The listing builds one solid part. Answer for the finished solid, in the listing's coordinates (mm). Face numbers are marked on the shaded views. A direction names the side the tool comes from. Give positions to 0.01 mm unless a question says otherwise; leave off trailing zeros. Write each loop counter-clockwise with the first axis right and the second up, starting at its lowest first coordinate (ties: lowest second). Pieces come first, ordered by that corner, then holes. Notation, with made-up numbers: (38, 69.5) - (97, 69.5) arc R8 ccw to (97, 79.5) - close; hole circle Ø2 at (45, 83.25). An arc over 180 degrees is marked (long way). Answer in a Markdown table with one row per item. Add a question column.
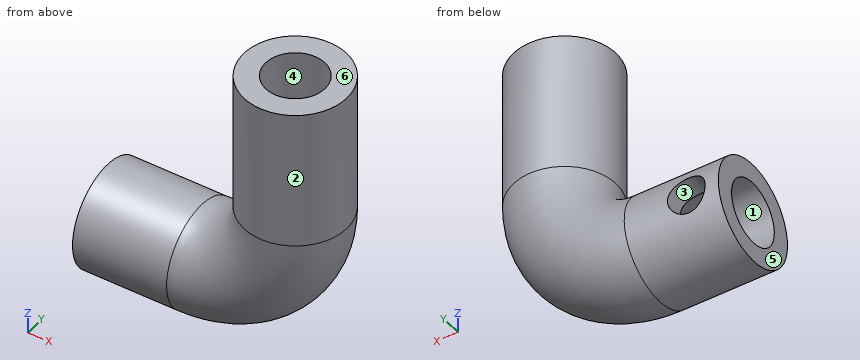
from build123d import *

# Parameters (mm, degrees)
SKETCH4_R         = 5.5
SKETCH6_R         = 3.175
HOLE_SHAFT_DEPTH  = 10
SKETCH7_R         = 3.4
HOLE_POT_DEPTH    = 10
SKETCH8_R         = 2
HOLE_INSERT_DEPTH = 6.5000001
SLOT_BOSS_DEPTH   = 1


with BuildPart() as part:
    # Sweep2: sweep along a path in PROFILE
    with BuildLine(Plane(origin=(0, 0, 0), x_dir=(1, 0, 0), z_dir=(0, 1, 0))) as sweep2_path:
        Line((2.5, -25), (2.5, -10))
        ThreePointArc((2.5, -10), (-0.428932188, -2.928932188), (-7.5, 0))
        Line((-7.5, 0), (-17.5, 0))
    # Sketch4 → Sweep2 (sweep)
    with BuildSketch(Plane.XY.offset(25)):
        with Locations((2.5, 0)):
            Circle(SKETCH4_R)
    sweep(path=sweep2_path.line)

    # Sketch6 → HOLE_SHAFT (cut)
    with BuildSketch(Plane.XY.offset(25)):
        with Locations((2.5, 0)):
            Circle(SKETCH6_R)
    extrude(amount=-HOLE_SHAFT_DEPTH, mode=Mode.SUBTRACT)

    # Sketch7 → HOLE_POT (cut)
    with BuildSketch(Plane.ZY.offset(17.5)):
        Circle(SKETCH7_R)
    extrude(amount=-HOLE_POT_DEPTH, mode=Mode.SUBTRACT)

    # Sketch8 → HOLE_INSERT (cut, through all)
    with BuildSketch(Plane(origin=(0, 0, 0), x_dir=(1, 0, 0), z_dir=(0, 1, 0))):
        with Locations((-14.096251262, 0)):
            Circle(SKETCH8_R)
    extrude(amount=HOLE_INSERT_DEPTH, mode=Mode.SUBTRACT)

    # Sketch11 → SLOT_BOSS (add)
    with BuildSketch(Plane.ZY.offset(7.5)):
        Polygon((1.645649924, -2.879269115), (-2.456130729, 2.466275506), (-1.662777389, 3.075036935), (2.439003264, -2.270507686), align=None)
    extrude(amount=SLOT_BOSS_DEPTH)


solid = part.part
1. Given pin 1 Ø2 at (y, z) = (0.5, -1.5) entering from -X; pin 2 Ø3 at (y, z) = (3, 16.5) entering from -X; pin 3 Ø5.5 at (x, y) = (2.5, 0) entering from +Z, each flat-ended and moving along its own axis, determine where each tip first touches the part or whether it passes through.
2. The mould has two halves that part along X. Classify the marked faces 4, 5 and 6: +X half, -X half, draft (parallel to the pull), parting line (faces both ways), or undercut.
3. A tool of negligible diameter and unlimited length cuts with its end or side. For the marked faces 1, 2 and 3, from which of +Z, -Z, +X, -X, +Y, -Y can it reach the whole face along a straight path? Write none if from no direction.
4. Section B-B (x = -9.25) is taken. Give the vertices of the cut face in (y, z).
5. Section A-A (y = 4.75) is taken. Give the vertices of the cut face in (x, z).
6. Section C-C (y = -4.5) is taken. Give the vertices of the cut face in (x, z).
7. Straight lines are drawn through the part: L1, parallel to Y at x = 2.5, z = 21 (3 decimals); L2, parallel to Y at x = -10.5, z = 0. For each, find the intervals that lie inside material, in ascending order. Write a range as [from, to].
8. Section D-D (z = 11) is taken. Give the vertices of the cut face in (x, y).
Geometry check:
| question | item | result |
|---|---|---|
| 1 | pin 1 | x = -8.5 |
| 1 | pin 2 | x = -2.79 |
| 1 | pin 3 | z = 15 |
| 2 | face 4 | undercut |
| 2 | face 5 | -X half |
| 2 | face 6 | draft |
| 3 | face 1 | -X |
| 3 | face 2 | +Z |
| 3 | face 3 | +Y |
| 4 | outline | circle Ø11 at (0, 0); hole circle Ø6.8 at (0, 0) |
| 5 | outline | (-17.5, -2.77) - (-7.5, -2.77) arc R12.77 ccw to (5.27, 10) - (5.27, 25) - (-0.27, 25) - (-0.27, 10) arc R7.23 cw to (-7.5, 2.77) - (-17.5, 2.77) - close; hole circle Ø4 at (-14.1, 0) |
| 6 | outline | (-17.5, -3.16) - (-7.5, -3.16) arc R13.16 ccw to (5.66, 10) - (5.66, 25) - (-0.66, 25) - (-0.66, 10) arc R6.84 cw to (-7.5, 3.16) - (-17.5, 3.16) - close |
| 7 | L1 | [-5.5, -3.175], [3.175, 5.5] |
| 7 | L2 | [-5.5, -3.4], [3.4, 5.5] |
| 8 | outline | circle Ø11 at (2.5, 0) |
